```python
from build123d import *

# Parameters (mm, degrees)
SKETCH_1_W      = 34.3
SKETCH_1_H      = 34.3
EXTRUDE_1_DEPTH = 2.5


with BuildPart() as part:
    # 草图1 → 凸台-拉伸1 (new body)
    with BuildSketch(Plane.XY):
        Rectangle(SKETCH_1_W, SKETCH_1_H)
        Polygon((6.531972647, 6.531972647), (-2.390867926, 8.922840573), (-8.922840573, 2.390867926), (-6.531972647, -6.531972647), (2.390867926, -8.922840573), (8.922840573, -2.390867926), align=None, mode=Mode.SUBTRACT)
    extrude(amount=EXTRUDE_1_DEPTH)


solid = part.part
```
CAD build for the part. Positions are in the model's coordinates, mm. A direction names the side the tool comes from. Round coordinates to 2 decimals unless told otherwise and drop trailing zeros. Order: outer loops, then holes, each group sorted by start corner. A loop starts at its lowest first (then second) coordinate and runs counter-clockwise, first axis right, second up. Notation, with made-up numbers: (-4, -8) - (37, -8) arc R16 cw to (37, 14) - close; hole circle Ø6 at (75.25, 54). An arc over 180 degrees is marked (long way). Use CSV: the item, a comma, the result in double quotes. Start each with the question number.
1) Saw through at A-A (z = 1.1). List the corners of the cut face in (x, y).
2) Tool access for faces 1 (the flat face through (-7.744, -2.008, 1.232)), 2 (the flat face through (0, -17.15, 1)): list every direction of +Z, -Z, +X, -X, +Y, -Y with a clear straight run to the whole face (end or side of a thin tool).
3) Saw through at B-B (y = 7.5). List the corners of the cut face in (x, z).
4) Saw through at C-C (x = 3). List the corners of the cut face in (y, z), and give its area (3 significant figures).
5) Two-plate mould, pull along Y, no slides. Class faces 3 (the flat face through (-8, 4, 2.5)), 4 (the flat face through (2.13, 7.71, 1.23)), 5 (the flat face through (0, 17.15, 1)): pulls with the +Y half, pulls with the -Y half, needs draft (parallel to the pull), parting line crosses it, or undercut.
6) Wall check: L1, parallel to X at y = 4, z = 2.35; L2, parallel to Y at x = -5, z = 2.25; L3, parallel to X at y = 3, z = 0.65. Give the ranges that are in metal, low to high. Write a range as [from, to].
Values follow:
1,outline,"(-17.15, -17.15) - (17.15, -17.15) - (17.15, 17.15) - (-17.15, 17.15) - close; hole (-8.92, 2.39) - (-6.53, -6.53) - (2.39, -8.92) - (8.92, -2.39) - (6.53, 6.53) - (-2.39, 8.92) - close"
2,face 1,"+Z, -Z"
2,face 2,"+Z, -Z, +X, -X, -Y"
3,outline,"(-17.15, 0) - (-3.81, 0) - (-3.81, 2.5) - (-17.15, 2.5) - close; (2.92, 0) - (17.15, 0) - (17.15, 2.5) - (2.92, 2.5) - close"
4,outline,"(-17.15, 0) - (-8.31, 0) - (-8.31, 2.5) - (-17.15, 2.5) - close; (7.48, 0) - (17.15, 0) - (17.15, 2.5) - (7.48, 2.5) - close"
4,area,"46.3 mm2"
5,face 3,"needs draft"
5,face 4,"undercut"
5,face 5,"pulls with the +Y half"
6,L1,"x = [-17.15, -7.31], [7.21, 17.15]"
6,L2,"y = [-17.15, -6.94], [6.31, 17.15]"
6,L3,"x = [-17.15, -8.31], [7.48, 17.15]"
